Autodesk Inventor part; units mm, degrees
ref_plane "YZ Plane" through (0, 0, 0) normal (1, 0, 0) x (0, 1, 0)
ref_plane "XZ Plane" through (0, 0, 0) normal (0, 1, 0) x (-1, 0, 0)
ref_plane "XY Plane" through (0, 0, 0) normal (0, 0, 1) x (1, 0, 0)
sketch "Sketch1" plane through (0, 0, 0) normal (0, 0, 1) x (1, 0, 0)
  line L0 (-20.5, 10) -> (20.5, 10)
  line L1 (20.5, 10) -> (20.5, -10)
  line L2 (20.5, -10) -> (-20.5, -10)
  line L3 (-20.5, -10) -> (-20.5, 10)
  line L4 (-20.5, 10) -> (20.5, -10) construction
  line L5 (20.5, 10) -> (-20.5, -10) construction
  circle A0 centre (6.5, 0) radius 2.5
  circle A1 centre (-6.5, 0) radius 2.5
  point P0 (0, 0)
  dimension "d0" = 41
  dimension "d1" = 20
  dimension "d2" = 5
  dimension "d3" = 6.5
  dimension "d4" = 5
  dimension "d5" = 6.5
extrude "Extrusion1" add sketch "Sketch1" along normal mid plane 0.5
properties part number "galvo spacer"
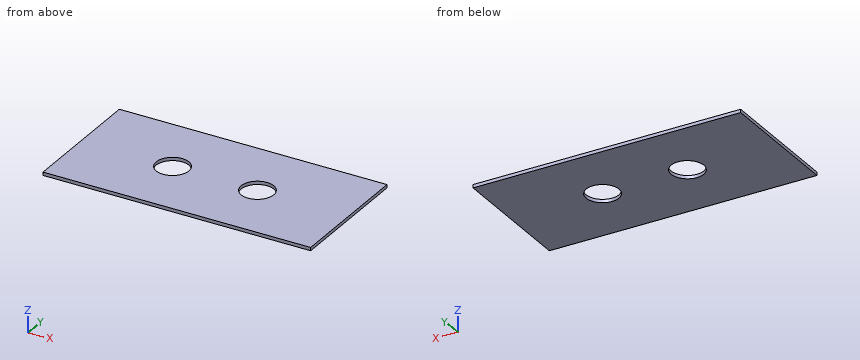
Can you work these out from the model? Positions are in its coordinate system, mm. Give positions to 0.01 mm unless a question says otherwise; leave off trailing zeros. Write each loop counter-clockwise with the first axis right and the second up, starting at its lowest first coordinate (ties: lowest second). Pieces come first, ordered by that corner, then holes. Notation, with made-up numbers: (-18, 72) -> (-3, 72) arc R23 cw to (-3, 104) -> close; hole circle Ø10 at (83, -28). An arc over 180 degrees is marked (long way). Answer as a JSON object with one key per item and string values. Group by question number.
Item 1: Suppose I cut it at B-B (x = -6.5). Please give me the cut outline in (y, z), plus the area to 3 significant figures.
Item 2: Suppose I cut it at C-C (z = 0.15). Please give me the cut outline in (x, y).
Item 3: I'm going to push a flat-ended pin straight in: P1, Ø6, axis at x = 6.5, y = 0, coming from the -Z side. Where does the tip first touch, or does it pass through?
Item 4: Suppose I cut it at A-A (y = 0). Please give me the cut outline in (x, z), plus the area to 3 significant figures.
Item 5: Please list where these lines run through material, in increasing order: line 1 (X direction, y = -2.25, z = 0.2); line 2 (Y direction, x = 6.5, z = 0.1); line 3 (X direction, y = 1.25, z = 0). Write a range as [from, to].
Findings:
{
 "1": {"outline": "(-10, -0.25) -> (-2.5, -0.25) -> (-2.5, 0.25) -> (-10, 0.25) -> close; (2.5, -0.25) -> (10, -0.25) -> (10, 0.25) -> (2.5, 0.25) -> close", "area": "7.50 mm²"},
 "2": {"outline": "(-20.5, -10) -> (20.5, -10) -> (20.5, 10) -> (-20.5, 10) -> close; hole circle Ø5 at (-6.5, 0); hole circle Ø5 at (6.5, 0)"},
 "3": {"P1": "stops at z = -0.25"},
 "4": {"outline": "(-20.5, -0.25) -> (-9, -0.25) -> (-9, 0.25) -> (-20.5, 0.25) -> close; (-4, -0.25) -> (4, -0.25) -> (4, 0.25) -> (-4, 0.25) -> close; (9, -0.25) -> (20.5, -0.25) -> (20.5, 0.25) -> (9, 0.25) -> close", "area": "15.5 mm²"},
 "5": {"line 1": "x = [-20.5, -7.59], [-5.41, 5.41], [7.59, 20.5]", "line 2": "y = [-10, -2.5], [2.5, 10]", "line 3": "x = [-20.5, -8.67], [-4.33, 4.33], [8.67, 20.5]"}
}
